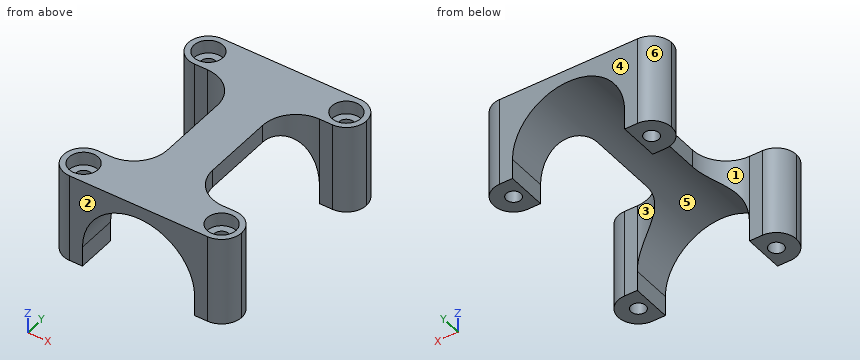
```python
from build123d import *

# Parameters (mm, degrees)
F1_DEPTH       = 49
F3_D           = 3.3
F3_DEPTH       = 30
F3_CBORE_D     = 6.5
F3_CBORE_DEPTH = 3
F3_TIP         = 0.9914200214
F5_DEPTH       = 25
F6_R           = 4.49999


# Not quite as in the source:
# - a fillet or chamfer is up to 0.001 mm smaller than in the source, because OpenCascade refuses the exact size


with BuildPart() as f1:
    # F0 (on Front) → F1 (new body)
    with BuildSketch(Plane.XZ):
        with BuildLine():
            Line((0, 20), (0, 0))
            Line((0, 0), (7.4, 0))
            Line((7.4, 0), (7.4, 4.5))
            ThreePointArc((7.4, 4.5), (20, 17.1), (32.6, 4.5))
            Line((32.6, 4.5), (32.6, 0))
            Line((32.6, 0), (40, 0))
            Line((40, 0), (40, 20))
            Line((40, 20), (0, 20))
        make_face()
    extrude(amount=F1_DEPTH)

    # F3
    with Locations(Plane.XY.offset(20)):
        with Locations((4.5, -4.5), (4.5, -44.5), (35.5, -44.5), (35.5, -4.5)):
            CounterBoreHole(F3_D / 2, F3_CBORE_D / 2, F3_CBORE_DEPTH, depth=F3_DEPTH)
            with Locations((0, 0, -(F3_DEPTH + F3_TIP / 2))):  # 118° drill point
                Cone(0, F3_D / 2, F3_TIP, mode=Mode.SUBTRACT)

    # F4 (on face) → F5 (cut)
    with BuildSketch(Plane.XY.offset(20)):
        with BuildLine():
            Line((14.9, -32.5), (14.9, -16.5))
            ThreePointArc((14.9, -16.5), (12.7033008589, -11.1966991411), (7.4, -9))
            Line((7.4, -9), (-0.1, -9))
            Line((-0.1, -9), (-0.1, -40))
            Line((-0.1, -40), (7.4, -40))
            ThreePointArc((7.4, -40), (12.7033008589, -37.8033008589), (14.9, -32.5))
        make_face()
        with BuildLine():
            ThreePointArc((32.6, -9), (27.2966991411, -11.1966991411), (25.1, -16.5))
            Line((25.1, -16.5), (25.1, -32.5))
            ThreePointArc((25.1, -32.5), (27.2966991411, -37.8033008589), (32.6, -40))
            Line((32.6, -40), (40.1, -40))
            Line((40.1, -40), (40.1, -9))
            Line((40.1, -9), (32.6, -9))
        make_face()
    extrude(amount=-F5_DEPTH, mode=Mode.SUBTRACT)

    # F6 (radius 4.5 in the source; OpenCascade refuses exactly that, so slightly less here)
    f6_edges = [f1.edges().sort_by_distance(p)[0] for p in [
        (40, -49, 10),
        (0, -49, 10),
        (40, 0, 10),
        (0, 0, 10),
        (40, -9, 10),
        (40, -40, 10),
        (0, -40, 10),
        (0, -9, 10),
    ]]
    fillet(f6_edges, radius=F6_R)


solid = f1.part
```
Part model, mm, in its own coordinate system. Face numbers are marked on the shaded views. A direction names the side the tool comes from. Round coordinates to 2 decimals unless told otherwise and drop trailing zeros. Order: outer loops, then holes, each group sorted by start corner. A loop starts at its lowest first (then second) coordinate and runs counter-clockwise, first axis right, second up. Notation, with made-up numbers: M 64.5,69 L 118.5,69 A24 ccw 118.5,100 Z; hole C 34.5,-36.75 d5. An arc over 180 degrees is marked long. Answer in a Markdown table with one row per item. Add a question column.
Q1. Pin check, flat tips, straight feed: pin 1 (2 mm diameter, centred on x = 35.5, y = -44.5, fed in from +Z); pin 2 (7 mm diameter, centred on x = 5.5, y = -44.5, fed in from +Z); pin 3 (2 mm diameter, centred on y = -46.5, z = 2, fed in from -X); pin 4 (5 mm diameter, centred on x = 36, y = -44, fed in from +Z). Stop position of each tip, or through.
Q2. Wall check: L1, parallel to Y at x = 35.5, z = 12; L2, parallel to Y at x = 4.5, z = 19.05; L3, parallel to X at y = -5, z = 18.5. Give the ranges that are in metal, low to high. Write a range as from..to.
Q3. Cut at B-B on x = 34.5. Give the cut face in (y, z).
Q4. Cut at A-A on z = 2. Give the number of separate pieces and of enclosed holes in the cut face, and give its area (3 significant figures).
Q5. Cut at C-C on y = -29. Give the cut face in (x, z), and give its area (3 significant figures).
Q6. 3-axis set-ups, long thin cutter, end or side, ignore diameter. For the marked faces 1, 2 and 3: which of +Z, -Z, +X, -X, +Y, -Y reach the whole face in a straight line?
Q7. Mould opens along X. For the marked faces 4, 5 and 6 say: +X half, -X half, draft (parallel to the pull), parting line (faces both ways), or undercut.
Established:
| question | item | result |
|---|---|---|
| 1 | pin 1 | passes through |
| 1 | pin 2 | stops at z = 20 |
| 1 | pin 3 | stops at x = 0.11 |
| 1 | pin 4 | stops at z = 17 |
| 2 | L1 | y = -49..-46.15, -42.85..-40, -9..-6.15, -2.85..0 |
| 2 | L2 | y = -49..-47.75, -41.25..-40, -9..-7.75, -1.25..0 |
| 2 | L3 | x = 0.03..1.29, 7.71..32.29, 38.71..39.97 |
| 3 | outline | M -49,0 L -45.81,0 L -45.81,17 L -47.59,17 L -47.59,20 L -49,20 Z; M -43.19,0 L -40,0 L -40,20 L -41.41,20 L -41.41,17 L -43.19,17 Z; M -9,0 L -5.81,0 L -5.81,17 L -7.59,17 L -7.59,20 L -9,20 Z; M -3.19,0 L 0,0 L 0,20 L -1.41,20 L -1.41,17 L -3.19,17 Z |
| 4 | separate pieces | 4 |
| 4 | enclosed holes | 4 |
| 4 | area | 197 mm2 |
| 5 | outline | M 14.9,16.02 A12.6 cw 25.1,16.02 L 25.1,20 L 14.9,20 Z |
| 5 | area | 33.2 mm2 |
| 6 | face 1 | +Z, -Z, -X |
| 6 | face 2 | +Z, -Z, +X, -X, -Y |
| 6 | face 3 | +Z, -Z, +X |
| 7 | face 4 | draft |
| 7 | face 5 | undercut |
| 7 | face 6 | -X half |
